Design review of the part built by this model. Coordinates are the model's own, in mm. Face numbers are marked on the shaded views. A direction names the side the tool comes from. Give positions to 0.01 mm unless a question says otherwise; leave off trailing zeros. Loops run counter-clockwise (first coordinate to the right, second up) from the corner with the lowest first, then second, coordinate; pieces in that order, holes last. Notation, with made-up numbers: M -25.75,27 L -7.75,27 A37 cw -7.75,64 Z; hole C 34,86 d2. An arc over 180 degrees is marked long. Use a Markdown table: item, result. Add a question column.
(1) Add section A-A, the plane z = 76. Give the boundary of the cut face in (x, y).
(2) Insertion check: pin 1 Ø3 at (x, y) = (57.5, 97.5) entering from +Z; pin 2 Ø18 at (x, y) = (49, 68) entering from +Z; pin 3 Ø4 at (x, y) = (28, 97.5) entering from +Z. Each pin has a flat end and moves straight along its axis. Give the tip position at first contact, or say it passes through.
(3) Draft analysis for pull direction Y (two halves, no side actions). For the marked faces 1, 2 and 3, state which applies: pulls with the +Y half, pulls with the -Y half, needs draft (parallel to the pull), parting line crosses it, or undercut.
(4) For probe 1 along X at (y, z) = (94, 22.5); probe 2 along X at (y, z) = (83, 18.5); probe 3 along Y at (x, z) = (57, 37), list the stretches that pass through material, from the lowest coordinate up.
(5) Add section C-C, the plane z = 35. Give the boundary of the cut face in (x, y).
(6) For the marked faces 4 and 5, list the 3-axis set-ups (+Z, -Z, +X, -X, +Y, -Y) from which the entire face can be reached by the end or side of a thin tool; tool diameter is ignored.
(7) Add section B-B, the plane y = 58. Give the boundary of the cut face in (x, z).
(8) Add section D-D, the plane x = 93. Give the boundary of the cut face in (y, z).
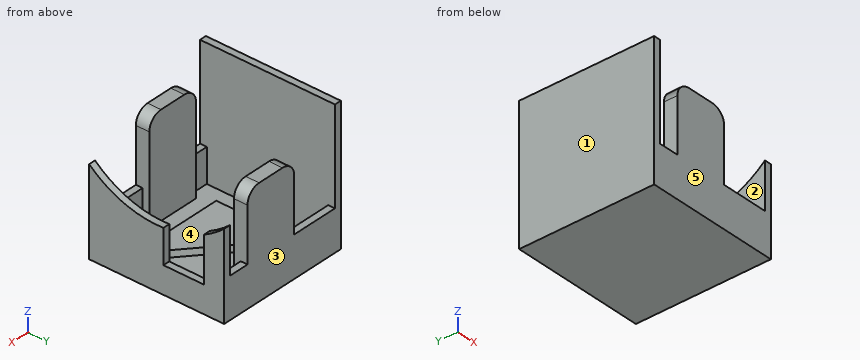
```python
from build123d import *

# Parameters (mm, degrees)
F0_W      = 100
F0_H      = 100
F1_DEPTH  = 5
F2_W      = 5
F2_H      = 100
F3_DEPTH  = 95
F5_DEPTH  = 5
F7_DEPTH  = 5
F9_DEPTH  = 5
F11_DEPTH = 5
F12_W     = 40
F12_H     = 5
F13_DEPTH = 75
F14_W     = 40
F14_H     = 5
F15_DEPTH = 75
F16_R     = 10


with BuildPart() as f1:
    # F0 (on Top) → F1 (new body)
    with BuildSketch(Plane.XY):
        with Locations((50, 50)):
            Rectangle(F0_W, F0_H)
    extrude(amount=F1_DEPTH)

    # F2 (on face) → F3 (join)
    with BuildSketch(Plane.XY.offset(5)):
        with Locations((2.5, 50)):
            Rectangle(F2_W, F2_H)
    extrude(amount=F3_DEPTH)

    # F4 (on face) → F5 (join)
    with BuildSketch(Plane.XY.offset(5)):
        Polygon((90, 25), (20, 85), (20, 25), align=None)
    extrude(amount=F5_DEPTH)

    # F6 (on face) → F7 (join)
    with BuildSketch(Plane.YZ.offset(100)):
        with BuildLine():
            Line((0, 64.098301), (0, 5))
            Line((0, 5), (100, 5))
            Line((100, 5), (100, 64.098301))
            ThreePointArc((100, 64.098301), (92.818809, 58.42444), (85, 53.667504))
            Line((85, 53.667504), (85, 20))
            Line((85, 20), (55, 20))
            Line((55, 20), (55, 45.166852))
            ThreePointArc((55, 45.166852), (25.589962, 49.083499), (0, 64.098301))
        make_face()
    extrude(amount=-F7_DEPTH)

    # F8 (on face) → F9 (join)
    with BuildSketch(Plane.XZ):
        Polygon((5, 30), (5, 5), (95, 5), (95, 30), (60, 30), (60, 80), (20, 80), (20, 30), align=None)
    extrude(amount=-F9_DEPTH)

    # F10 (on face) → F11 (join)
    with BuildSketch(Plane(origin=(0, 100, 0), x_dir=(-1, 0, 0), z_dir=(0, 1, 0))):
        Polygon((-95, 5), (-5, 5), (-5, 30), (-40, 30), (-40, 80), (-80, 80), (-80, 30), (-95, 30), align=None)
    extrude(amount=-F11_DEPTH)

    # F12 (on face) → F13 (join, through all)
    with BuildSketch(Plane.XY.offset(80)):
        with Locations((40, 7.5)):
            Rectangle(F12_W, F12_H)
    extrude(amount=-F13_DEPTH)

    # F14 (on face) → F15 (join, through all)
    with BuildSketch(Plane.XY.offset(80)):
        with Locations((60, 92.5)):
            Rectangle(F14_W, F14_H)
    extrude(amount=-F15_DEPTH)

    # F16
    f16_edges = [f1.edges().sort_by_distance(p)[0] for p in [
        (60, 5, 80),
        (20, 5, 80),
        (80, 95, 80),
        (40, 95, 80),
    ]]
    fillet(f16_edges, radius=F16_R)


solid = f1.part
```
Established:
| question | item | result |
|---|---|---|
| 1 | outline | M 0,0 L 5,0 L 5,100 L 0,100 Z; M 22,0 L 58,0 L 58,10 L 22,10 Z; M 42,90 L 78,90 L 78,100 L 42,100 Z |
| 2 | pin 1 | z = 80 |
| 2 | pin 2 | z = 10 |
| 2 | pin 3 | z = 30 |
| 3 | face 1 | needs draft |
| 3 | face 2 | undercut |
| 3 | face 3 | pulls with the +Y half |
| 4 | probe 1 | 0 to 5, 40 to 80, 95 to 100 |
| 4 | probe 2 | 0 to 5, 95 to 100 |
| 4 | probe 3 | 0 to 10, 90 to 100 |
| 5 | outline | M 0,0 L 5,0 L 5,100 L 0,100 Z; M 20,0 L 60,0 L 60,10 L 20,10 Z; M 40,90 L 80,90 L 80,100 L 40,100 Z; M 95,0 L 100,0 L 100,55 L 95,55 Z; M 95,85 L 100,85 L 100,100 L 95,100 Z |
| 6 | face 4 | +Z |
| 6 | face 5 | +Z, -Z, +X, -X, -Y |
| 7 | outline | M 0,0 L 100,0 L 100,20 L 95,20 L 95,5 L 51.5,5 L 51.5,10 L 20,10 L 20,5 L 5,5 L 5,100 L 0,100 Z |
| 8 | outline | M 0,0 L 100,0 L 100,30 L 95,30 L 95,5 L 5,5 L 5,30 L 0,30 Z |
